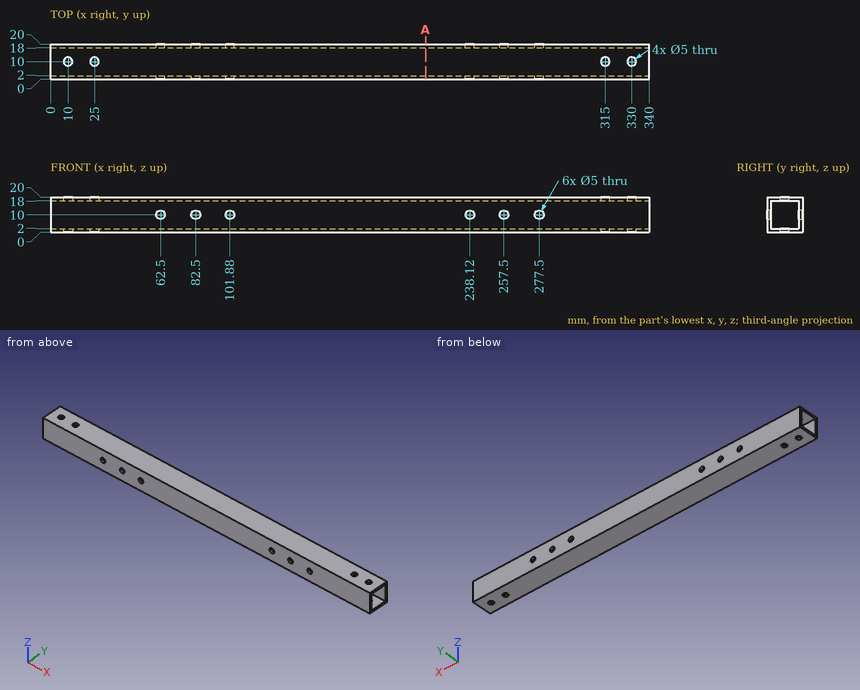
Could you check a few things on this drawing? It's one solid part, dimensions in mm from its lowest x, y, z. Give positions to 0.01 mm unless a question says otherwise; leave off trailing zeros. Loops run counter-clockwise (first coordinate to the right, second up) from the corner with the lowest first, then second, coordinate; pieces in that order, holes last. Notation, with made-up numbers: (70, 49) -> (90, 49) arc R16 ccw to (90, 74) -> close; hole circle Ø6 at (-11, 5). An arc over 180 degrees is marked (long way). Answer as CSV lines item,"result". Start each with the question number.
(1) If we section it at A-A on x = 213: Write out the boundary of the cut face in (y, z), then the cut area to 3 significant figures.
(2) I need wall thicknesses on probe 1 along Z at (x, y) = (208.5, 5.25); probe 2 along Z at (x, y) = (238.12, 1). Which ranges of each line are inside material? Lowest first, please.
(3) I'm going to push flat-ended pins straight in: pin 1 Ø4 at (x, y) = (330, 10) entering from -Z; pin 2 Ø6 at (x, z) = (238.12, 10) entering from -Y. Where does each tip first touch, or does it pass through?
Computed:
1,outline,"(0, 0) -> (20, 0) -> (20, 20) -> (0, 20) -> close; hole (2, 2) -> (18, 2) -> (18, 18) -> (2, 18) -> close"
1,area,"144 mm2"
2,probe 1,"z = 0 to 2, 18 to 20"
2,probe 2,"z = 0 to 7.5, 12.5 to 20"
3,pin 1,"passes through"
3,pin 2,"stops at y = 0"
